from build123d import *

# Parameters (mm, degrees)
MAIN_DEPTH                  = 5.13
SKETCH2_W                   = 16.6
SKETCH2_H                   = 5.13
TEETH_DEPTH                 = 5.13
M3_CLEARANCE_HOLE1_D        = 3.2
M3_CLEARANCE_HOLE1_DEPTH    = 5.13
HINGE_SLOT_REACH            = 7.13
THERMISTOR_WIRES_HOLE_REACH = 7.13
SKETCH6_R                   = 3.175


with BuildPart() as part:
    # Sketch1 → Main (new body)
    with BuildSketch(Plane.XY):
        with BuildLine():
            Line((-56.488759744, 30.356747088), (41.871240256, 30.356747088))
            Line((41.871240256, 30.356747088), (41.871240256, 2.356747088))
            ThreePointArc((41.871240256, 2.356747088), (41.578347037, 1.649640307), (40.871240256, 1.356747088))
            Line((40.871240256, 1.356747088), (-55.488759744, 1.356747088))
            ThreePointArc((-55.488759744, 1.356747088), (-56.195866525, 1.649640307), (-56.488759744, 2.356747088))
            Line((-56.488759744, 2.356747088), (-56.488759744, 30.356747088))
        make_face()
    extrude(amount=MAIN_DEPTH)

    # Sketch2 → Teeth (add)
    with BuildSketch(Plane(origin=(0, 30.356747088, 0), x_dir=(1, 0, 0), z_dir=(0, 1, 0))):
        with Locations((9.291240256, -2.565)):
            Rectangle(SKETCH2_W, SKETCH2_H)
        with Locations((-23.908759744, -2.565)):
            Rectangle(SKETCH2_W, SKETCH2_H)
    extrude(amount=TEETH_DEPTH)

    # M3 Clearance Hole1
    with Locations(Plane.XY.offset(5.13)):
        with Locations((-46.923759744, 16.856747088), (32.306240256, 16.856747088)):
            Hole(M3_CLEARANCE_HOLE1_D / 2, depth=M3_CLEARANCE_HOLE1_DEPTH)

    # Sketch5 → Hinge slot (cut, up to next)
    with BuildSketch(Plane.XY.offset(5.13), mode=Mode.PRIVATE) as hinge_slot_sk1:
        with BuildLine():
            Line((-29.168759744, 26.356747088), (14.551240256, 26.356747088))
            ThreePointArc((14.551240256, 26.356747088), (15.258347037, 26.06385387), (15.551240256, 25.356747088))
            Line((15.551240256, 25.356747088), (15.551240256, 1.356747088))
            Line((15.551240256, 1.356747088), (-30.168759744, 1.356747088))
            Line((-30.168759744, 1.356747088), (-30.168759744, 25.356747088))
            ThreePointArc((-30.168759744, 25.356747088), (-29.875866525, 26.06385387), (-29.168759744, 26.356747088))
        make_face()
    hinge_slot_tool1 = extrude(hinge_slot_sk1.sketch, amount=-HINGE_SLOT_REACH, mode=Mode.PRIVATE) & part.part
    add(hinge_slot_tool1.solids().sort_by_distance((-7.30876, 13.852135, 5.13))[0], mode=Mode.SUBTRACT)

    # Sketch6 → Thermistor wires hole (cut, up to next)
    with BuildSketch(Plane.XY.offset(5.13), mode=Mode.PRIVATE) as thermistor_wires_hole_sk1:
        with Locations((28.738240256, 12.652139603)):
            Circle(SKETCH6_R)
    thermistor_wires_hole_tool1 = extrude(thermistor_wires_hole_sk1.sketch, amount=-THERMISTOR_WIRES_HOLE_REACH, mode=Mode.PRIVATE) & part.part
    add(thermistor_wires_hole_tool1.solids().sort_by_distance((28.73824, 12.65214, 5.13))[0], mode=Mode.SUBTRACT)


solid = part.part
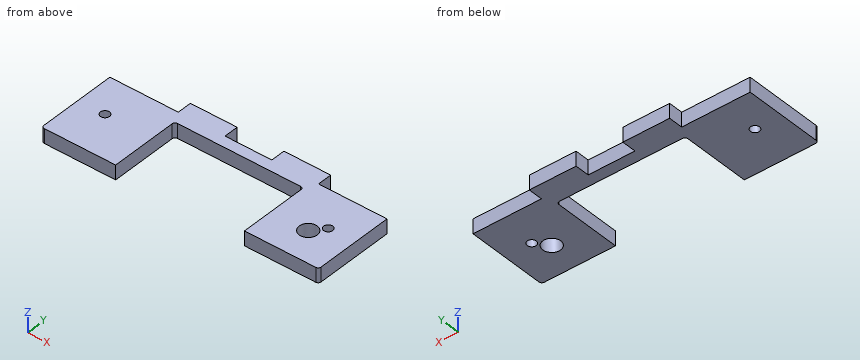
The listing builds one solid part. Answer for the finished solid, in the listing's coordinates (mm). Coordinates: 2 decimals unless noted, no trailing zeros. Order: outer loops, then holes, each group sorted by start corner. A loop starts at its lowest first (then second) coordinate and runs counter-clockwise, first axis right, second up.
Q1. Given P1, Ø1, axis at x = -37, y = 21, coming from the -Z side; P2, Ø1.5, axis at x = 2.5, z = 2, coming from the -Y side; P3, Ø2.5, axis at x = -46.5, z = 2, coming from the +Y side; P4, Ø1.5, axis at y = 32, z = 3.5, coming from the -X side, each flat-ended and moving along its own axis, determine where each tip first touches the part or whether it passes through.
Q2. A cutting plane is placed at A-A, the plane y = 23. Write down the section's boundary in (x, z), and give its area (3 significant figures).
Q3. A cutting plane is placed at B-B, the plane z = 2.8. Write down the section's boundary in (x, y) (3 decimals).
Q4. Consider line 1 (X direction, y = 22.5, z = 0.95); line 2 (X direction, y = 33.5, z = 3.9); line 3 (X direction, y = 10, z = 4.35). Determine where each line is inside the solid, lowest interval first.
Q5. A cutting plane is placed at D-D, the plane x = 8. Write down the section's boundary in (y, z), and give its area (3 significant figures).
Q6. A cutting plane is placed at C-C, the plane x = 24. Write down the section's boundary in (y, z), and give its area (3 significant figures).
Answers follow:
1. P1: stops at z = 0
1. P2: stops at y = 26.36
1. P3: stops at y = 30.36
1. P4: stops at x = -32.21
2. outline: (-56.49, 0) - (-30.17, 0) - (-30.17, 5.13) - (-56.49, 5.13) - close; (15.55, 0) - (41.87, 0) - (41.87, 5.13) - (15.55, 5.13) - close
2. area: 270 mm2
3. outline: (-56.489, 2.357) arc R1 ccw to (-55.489, 1.357) - (-30.169, 1.357) - (-30.169, 25.357) arc R1 cw to (-29.169, 26.357) - (14.551, 26.357) arc R1 cw to (15.551, 25.357) - (15.551, 1.357) - (40.871, 1.357) arc R1 ccw to (41.871, 2.357) - (41.871, 30.357) - (17.591, 30.357) - (17.591, 35.487) - (0.991, 35.487) - (0.991, 30.357) - (-15.609, 30.357) - (-15.609, 35.487) - (-32.209, 35.487) - (-32.209, 30.357) - (-56.489, 30.357) - close; hole circle Ø3.2 at (-46.924, 16.857); hole circle Ø6.35 at (28.738, 12.652); hole circle Ø3.2 at (32.306, 16.857)
4. line 1: x = -56.49 to -30.17, 15.55 to 41.87
4. line 2: x = -32.21 to -15.61, 0.99 to 17.59
4. line 3: x = -56.49 to -30.17, 15.55 to 26.99, 30.48 to 41.87
5. outline: (26.36, 0) - (35.49, 0) - (35.49, 5.13) - (26.36, 5.13) - close
5. area: 46.8 mm2
6. outline: (1.36, 0) - (30.36, 0) - (30.36, 5.13) - (1.36, 5.13) - close
6. area: 149 mm2
